from build123d import *

# Parameters (mm, degrees)
EXTRUDE_1_DEPTH             = 6
CUT_EXTRUDE_1_DEPTH         = 7
HOLE_WIZARD_M24_1_D         = 27
HOLE_WIZARD_M24_1_DEPTH     = 6
HOLE_WIZARD_10_0_10_1_D     = 10
HOLE_WIZARD_10_0_10_1_DEPTH = 6
HOLE_WIZARD_3_2_3_2_1_D     = 3.2
HOLE_WIZARD_3_2_3_2_1_DEPTH = 6
FILLET_1_R                  = 5
CHAMFER_1_SIZE              = 0.5


with BuildPart() as part:
    # 草图1 → 凸台-拉伸1 (new body)
    with BuildSketch(Plane.XY.offset(6)):
        with BuildLine():
            Line((-50.844308234, -26.095570892), (-51.795328938, -30.582125502))
            ThreePointArc((-51.795328938, -30.582125502), (42.532472888, -42.532472888), (30.582125502, 51.795328938))
            Line((30.582125502, 51.795328938), (26.095570892, 50.844308234))
            ThreePointArc((26.095570892, 50.844308234), (-40.411152545, 40.411152545), (-50.844308234, -26.095570892))
        make_face()
    extrude(amount=-EXTRUDE_1_DEPTH)

    # 草图2 → 切除-拉伸1 (cut, through all)
    with BuildSketch(Plane(origin=(0, 0, 0), x_dir=(-1, 0, 0), z_dir=(0, 0, -1))):
        with BuildLine():
            Line((30.582125502, -51.795328938), (26.095570892, -50.844308234))
            ThreePointArc((26.095570892, -50.844308234), (-40.411152545, -40.411152545), (-50.844308234, 26.095570892))
            Line((-50.844308234, 26.095570892), (-51.795328938, 30.582125502))
            ThreePointArc((-51.795328938, 30.582125502), (-42.532472888, -42.532472888), (30.582125502, -51.795328938))
        make_face()
    extrude(amount=-CUT_EXTRUDE_1_DEPTH, mode=Mode.SUBTRACT)

    # M24 间隙孔1
    with Locations(Plane(origin=(0, 0, 0), x_dir=(-1, 0, 0), z_dir=(0, 0, -1))):
        with Locations((0, -20)):
            Hole(HOLE_WIZARD_M24_1_D / 2, depth=HOLE_WIZARD_M24_1_DEPTH)

    # Ø10.0 (10) 直径孔1
    with Locations(Plane(origin=(0, 0, 0), x_dir=(-1, 0, 0), z_dir=(0, 0, -1))):
        with Locations((0, 30), (-30, 0), (30, 0)):
            Hole(HOLE_WIZARD_10_0_10_1_D / 2, depth=HOLE_WIZARD_10_0_10_1_DEPTH)

    # Ø3.2 (3.2) 直径孔1
    with Locations(Plane(origin=(0, 0, 0), x_dir=(-1, 0, 0), z_dir=(0, 0, -1))):
        with Locations((38.166088515, 38.166088515), (13.969757959, -52.135846474), (-13.969757959, 52.135846474), (-52.135846474, 13.969757959), (-38.166088515, -38.166088515), (52.135846474, -13.969757959)):
            Hole(HOLE_WIZARD_3_2_3_2_1_D / 2, depth=HOLE_WIZARD_3_2_3_2_1_DEPTH)

    # 圆角1
    fillet_1_edges = [part.edges().sort_by_distance(p)[0] for p in [
        (-30.582125502, -51.795328938, 3),
        (51.795328938, 30.582125502, 3),
        (50.844308234, 26.095570892, 3),
        (-26.095570892, -50.844308234, 3),
        (26.095570892, 50.844308234, 3),
        (30.582125502, 51.795328938, 3),
        (-51.795328938, -30.582125502, 3),
        (-50.844308234, -26.095570892, 3),
    ]]
    fillet(fillet_1_edges, radius=FILLET_1_R)

    # 倒角1
    chamfer_1_edges = [part.edges().sort_by_distance(p)[0] for p in [
        (51.409995233, 30.560581919, 0),
        (-30.560581919, -51.409995233, 0),
        (30.560581919, 51.409995233, 0),
        (-26.167497672, -51.130344697, 0),
        (51.130344697, 26.167497672, 0),
        (26.167497672, 51.130344697, 0),
        (-51.130344697, -26.167497672, 0),
        (40.411152545, -40.411152545, 0),
        (-28.212098099, -51.292951206, 0),
        (42.532472888, 42.532472888, 0),
        (28.212098099, 51.292951206, 0),
        (51.292951206, 28.212098099, 0),
        (-42.532472888, -42.532472888, 0),
        (-51.292951206, -28.212098099, 0),
        (-40.411152545, 40.411152545, 0),
        (-51.409995233, -30.560581919, 0),
    ]]
    chamfer(chamfer_1_edges, length=CHAMFER_1_SIZE)


solid = part.part
Here's how the part is built. I have some questions about the finished solid (model axes, mm). Round coordinates to 2 decimals unless told otherwise and drop trailing zeros. Loops run counter-clockwise (first coordinate to the right, second up) from the corner with the lowest first, then second, coordinate; pieces in that order, holes last. Notation, with made-up numbers: M 34.5,-13.5 L 90.5,-13.5 A36 cw 90.5,22.5 Z; hole C 75,-25.5 d8. An arc over 180 degrees is marked long. Write each question's results on one line, items separated by ' | '. Start each with the question number.
(1) If I drill on probe 1 along Y at (x, z) = (0, 2.55); probe 2 along X at (y, z) = (-2.5, 4); probe 3 along Y at (x, z) = (38.5, 5.75), over which ranges is the centre line in solid material (lowest first)? Write a range as from..to.
(2) I want a section at B-B (x = 0). Please give me the cut outline in (y, z), then the cut area to 3 significant figures.
(3) Will these pins go through, and if not, where does the flat tip stop? P1, Ø2, axis at y = 34, z = 3, coming from the -X side; P2, Ø16, axis at x = 0, y = -20, coming from the -Z side; P3, Ø2, axis at x = -21, z = 5, coming from the -Y side.
(4) I want a section at C-C (z = 4). State how many separate pieces and enclosed holes the cut face has, then the cut area to 3 significant figures.
(5) I want a section at A-A (y = 0). Please give me the cut outline in (x, z).
(6) Thinking about a two-plate mould opening in X: for faces 1 (the cylindrical face through (51.405, 30.587, 3.288)), 2 (the flat face through (-1, 1, 6)), 3 (the cylindrical face through (30.534, 51.415, 3.212)), which applies, pulls with the +X half, pulls with the -X half, needs draft (parallel to the pull), parting line crosses it, or undercut?
Solved:
1) probe 1: y = -57.15..-33.5, -6.5..25, 35..57.15 | probe 2: x = -57.1..-34.33, -25.67..25.67, 34.33..57.1 | probe 3: y = -42.24..-39.73, -36.6..46.21
2) outline: M -57.15,0.5 L -56.65,0 L -33.5,0 L -33.5,6 L -57.15,6 Z; M -6.5,0 L 25,0 L 25,6 L -6.5,6 Z; M 35,0 L 56.65,0 L 57.15,0.5 L 57.15,6 L 35,6 Z | area: 464 mm²
3) P1: stops at x = -46.66 | P2: passes through | P3: stops at y = -53.54
4) separate pieces: 1 | enclosed holes: 10 | area: 9,600 mm²
5) outline: M -57.15,0.5 L -56.65,0 L -35,0 L -35,6 L -57.15,6 Z; M -25,0 L 25,0 L 25,6 L -25,6 Z; M 35,0 L 56.65,0 L 57.15,0.5 L 57.15,6 L 35,6 Z
6) face 1: pulls with the +X half | face 2: needs draft | face 3: undercut
